Source: CAD feature listing. Evaluate the final solid. Frame: model axes, mm. A direction names the side the tool comes from. Coordinates: 2 decimals unless noted, no trailing zeros. Order: outer loops, then holes, each group sorted by start corner. A loop starts at its lowest first (then second) coordinate and runs counter-clockwise, first axis right, second up. Notation, with made-up numbers: (85.5, 9.5) - (116.5, 9.5) arc R28 ccw to (116.5, 47.5) - close; hole circle Ø6 at (-24.5, 70.25). An arc over 180 degrees is marked (long way). One line per question, with ' | ' between items. Start each with the question number.
(1) Line query: line 1 along X through (y, z) = (6.5, -0.2); line 2 along X through (y, z) = (4.5, 1.4); line 3 along Y through (x, z) = (5, 0.3). Output: solid intervals per line, ascending.
(2) Section B-B (y = 0). Return the cut outline in (x, z).
(3) Section A-A (x = 0). Return the cut outline in (y, z).
(4) Contact query for flat-ended pins moving along their axis: P1, Ø1, axis at x = 2, z = -1.5, coming from the -Y side; P2, Ø1.2, axis at y = 2, z = 0.5, coming from the +X side; P3, Ø2, axis at x = 12.5, z = -1.5, coming from the +Y side. Output: stop coordinate, or through.
(5) Access query for faces 1 (the flat face through (-6.8, 0, 0)), 2 (the flat face through (7, 0, -2)). Directions: +Z, -Z, +X, -X, +Y, -Y. A direction counts if a zero-diameter tool reaches every point of the face in a straight line with its end or side. Return the directions, or none.
from build123d import *

# Parameters (mm, degrees)
SKETCH_1_R      = 17.5
EXTRUDE_2_DEPTH = 2
CHAMFER_1_SIZE  = 0.5
FILLET_2_R      = 0.5


with BuildPart() as part:
    # Эскиз1 → Бобышка-Вытянуть2 (new, symmetric)
    with BuildSketch(Plane.XY):
        Circle(SKETCH_1_R)
        with BuildLine():
            Line((6.8, 4.308421985), (6.8, -4.308421985))
            ThreePointArc((6.8, -4.308421985), (0, -8.05), (-6.8, -4.308421985))
            Line((-6.8, -4.308421985), (-6.8, 4.308421985))
            ThreePointArc((-6.8, 4.308421985), (0, 8.05), (6.8, 4.308421985))
        make_face(mode=Mode.SUBTRACT)
    extrude(amount=EXTRUDE_2_DEPTH, both=True)

    # Эскиз2 → Вырез-Повернуть1 (revolve, cut)
    with BuildSketch(Plane(origin=(0, 0, 0), x_dir=(0, 0, -1), z_dir=(1, 0, 0)), mode=Mode.PRIVATE) as cut_revolve_1_sk:
        Polygon((-0.577350269, 17.5), (0.577350269, 17.5), (0, 16.5), align=None)
    revolve(cut_revolve_1_sk.sketch.rotate(Axis((0, 0, 3.24866267), (0, 0, -1)), 90), axis=Axis((0, 0, 3.24866267), (0, 0, -1)), mode=Mode.SUBTRACT)

    # Фаска1
    chamfer_1_edges = [part.edges().sort_by_distance(p)[0] for p in [
        (-17.5, 0, 2),
    ]]
    chamfer(chamfer_1_edges, length=CHAMFER_1_SIZE)

    # Скругление2
    fillet_2_edges = [part.edges().sort_by_distance(p)[0] for p in [
        (-17.5, 0, -2),
    ]]
    fillet(fillet_2_edges, radius=FILLET_2_R)


solid = part.part
Response values:
1) line 1: x = -15.54 to -4.75, 4.75 to 15.54 | line 2: x = -16.91 to -6.67, 6.67 to 16.91 | line 3: y = -16.27 to -6.31, 6.31 to 16.27
2) outline: (-17.5, -1.5) arc R0.5 ccw to (-17, -2) - (-6.8, -2) - (-6.8, 2) - (-17, 2) - (-17.5, 1.5) - (-17.5, 0.58) - (-16.5, 0) - (-17.5, -0.58) - close; (6.8, -2) - (17, -2) arc R0.5 ccw to (17.5, -1.5) - (17.5, -0.58) - (16.5, 0) - (17.5, 0.58) - (17.5, 1.5) - (17, 2) - (6.8, 2) - close
3) outline: (-17.5, -1.5) arc R0.5 ccw to (-17, -2) - (-8.05, -2) - (-8.05, 2) - (-17, 2) - (-17.5, 1.5) - (-17.5, 0.58) - (-16.5, 0) - (-17.5, -0.58) - close; (8.05, -2) - (17, -2) arc R0.5 ccw to (17.5, -1.5) - (17.5, -0.58) - (16.5, 0) - (17.5, 0.58) - (17.5, 1.5) - (17, 2) - (8.05, 2) - close
4) P1: stops at y = -17.44 | P2: stops at x = 17.44 | P3: stops at y = 13.19
5) face 1: +Z, -Z | face 2: -Z, +X, -X, +Y, -Y
